```python
from build123d import *

# Parameters (mm, degrees)
F3_W         = 27
F3_H         = 27
F4_DEPTH     = 30
F5_T1_DEPTH  = 1002
F5_T3_DEPTH  = 1038
F5_T5_DEPTH  = 442
F5_T7_DEPTH  = 478
F5_T13_DEPTH = 447
F5_T17_DEPTH = 1007
F5_T20_DEPTH = 1012
F5_T22_DEPTH = 1050
F5_T24_DEPTH = 1005
F5_T26_DEPTH = 445
F5_T28_DEPTH = 490
F5_T30_DEPTH = 452
F5_T36_DEPTH = 1010
F5_T40_DEPTH = 450
F5_T47_DEPTH = 1010
F5_T51_DEPTH = 450


# Not quite as in the source:
# - a fillet or chamfer that OpenCascade refuses, or shapes differently, is made with other operations: its cross-section is extruded or revolved along the edge and cut away or added


with BuildPart() as f2:
    # F2: sweep along a path in F1
    with BuildLine(Plane.XY) as f2_path:
        Line((0, 0), (0, 440))
        Line((0, 440), (-1000, 440))
    # F0 (on Front) → F2 (sweep)
    with BuildSketch(Plane.XZ):
        Polygon((38, -2), (38, -25), (40, -25), (40, 0), (0, 0), (0, -350), (27, -350), (27, -376), (29, -376), (29, -348), (2, -348), (2, -2), align=None)
    sweep(path=f2_path.line, transition=Transition.RIGHT)

    # F3 (on face) → F4 (cut)
    with BuildSketch(Plane.XY.offset(-348)):
        with Locations((15.5, 455.5)):
            Rectangle(F3_W, F3_H)
    extrude(amount=-F4_DEPTH, mode=Mode.SUBTRACT)

    # F5: fillet of radius 2 on 15 edges, made by hand

    # F5_s2 → F5_t1 (join)
    with BuildSketch(Plane.YZ.offset(-1000)):
        with BuildLine():
            ThreePointArc((442, -346), (442.5857864376, -347.4142135624), (444, -348))
            Line((444, -348), (442, -348))
            Line((442, -348), (442, -346))
        make_face()
        with BuildLine():
            ThreePointArc((465, -350), (466.4142135624, -350.5857864376), (467, -352))
            Line((467, -352), (467, -350))
            Line((467, -350), (465, -350))
        make_face()
        with BuildLine():
            ThreePointArc((444, -2), (442.5857864376, -2.5857864376), (442, -4))
            Line((442, -4), (442, -2))
            Line((442, -2), (444, -2))
        make_face()
    extrude(amount=F5_T1_DEPTH)

    # F5_s4 → F5_t3 (join)
    with BuildSketch(Plane.YZ.offset(-1000)):
        with BuildLine():
            ThreePointArc((476, -2), (477.4142135624, -2.5857864376), (478, -4))
            Line((478, -4), (478, -2))
            Line((478, -2), (476, -2))
        make_face()
    extrude(amount=F5_T3_DEPTH)

    # F5_s6 → F5_t5 (join)
    with BuildSketch(Plane.XZ.offset(-442)):
        with BuildLine():
            ThreePointArc((25, -350), (26.4142135624, -350.5857864376), (27, -352))
            Line((27, -352), (27, -350))
            Line((27, -350), (25, -350))
        make_face()
        with BuildLine():
            ThreePointArc((4, -2), (2.5857864376, -2.5857864376), (2, -4))
            Line((2, -4), (2, -2))
            Line((2, -2), (4, -2))
        make_face()
    extrude(amount=F5_T5_DEPTH)

    # F5_s8 → F5_t7 (join)
    with BuildSketch(Plane.XZ.offset(-478)):
        with BuildLine():
            ThreePointArc((38, -4), (37.4142135624, -2.5857864376), (36, -2))
            Line((36, -2), (38, -2))
            Line((38, -2), (38, -4))
        make_face()
    extrude(amount=F5_T7_DEPTH)


with BuildPart() as f5_tool11:
    # F5_s12 → F5_t13 (new body)
    with BuildSketch(Plane.XZ):
        with BuildLine():
            ThreePointArc((4, -2), (2.5857864376, -2.5857864376), (2, -4))
            Line((2, -4), (2, -2))
            Line((2, -2), (4, -2))
        make_face()
    extrude(amount=-F5_T13_DEPTH)

    split(bisect_by=Plane.XZ.offset(-442), keep=Keep.BOTTOM)


with BuildPart() as f5_tool15:
    # F5_s16 → F5_t17 (new body)
    with BuildSketch(Plane.YZ.offset(7)):
        with BuildLine():
            ThreePointArc((444, -2), (442.5857864376, -2.5857864376), (442, -4))
            Line((442, -4), (442, -2))
            Line((442, -2), (444, -2))
        make_face()
    extrude(amount=-F5_T17_DEPTH)

    split(bisect_by=Plane.YZ.offset(2), keep=Keep.TOP)


with BuildPart() as f5_tool11_1:
    add(f5_tool11.part)

    # F5_t19: intersect F5_tool15
    add(f5_tool15.part, mode=Mode.INTERSECT)


with BuildPart() as f2_1:
    add(f2.part)

    # F5_t9: union F5_tool11
    add(f5_tool11_1.part)

    # F5_s21 → F5_t20 (cut)
    with BuildSketch(Plane.YZ.offset(-1005)):
        with BuildLine():
            ThreePointArc((467, -348), (468.4142135624, -348.5857864376), (469, -350))
            Line((469, -350), (469, -348))
            Line((469, -348), (467, -348))
        make_face()
    extrude(amount=F5_T20_DEPTH, mode=Mode.SUBTRACT)

    # F5_s23 → F5_t22 (cut)
    with BuildSketch(Plane.YZ.offset(-1005)):
        with BuildLine():
            ThreePointArc((480, -2), (479.4142135624, -0.5857864376), (478, 0))
            Line((478, 0), (480, 0))
            Line((480, 0), (480, -2))
        make_face()
    extrude(amount=F5_T22_DEPTH, mode=Mode.SUBTRACT)

    # F5_s25 → F5_t24 (cut)
    with BuildSketch(Plane.YZ.offset(-1005)):
        with BuildLine():
            ThreePointArc((440, -2), (440.5857864376, -0.5857864376), (442, 0))
            Line((442, 0), (440, 0))
            Line((440, 0), (440, -2))
        make_face()
        with BuildLine():
            ThreePointArc((440, -348), (440.5857864376, -349.4142135624), (442, -350))
            Line((442, -350), (440, -350))
            Line((440, -350), (440, -348))
        make_face()
    extrude(amount=F5_T24_DEPTH, mode=Mode.SUBTRACT)

    # F5_s27 → F5_t26 (cut)
    with BuildSketch(Plane.XZ.offset(-440)):
        with BuildLine():
            ThreePointArc((0, -2), (0.5857864376, -0.5857864376), (2, 0))
            Line((2, 0), (0, 0))
            Line((0, 0), (0, -2))
        make_face()
        with BuildLine():
            ThreePointArc((2, -350), (0.5857864376, -349.4142135624), (0, -348))
            Line((0, -348), (0, -350))
            Line((0, -350), (2, -350))
        make_face()
    extrude(amount=F5_T26_DEPTH, mode=Mode.SUBTRACT)

    # F5_s29 → F5_t28 (cut)
    with BuildSketch(Plane.XZ.offset(-485)):
        with BuildLine():
            ThreePointArc((38, 0), (39.4142135624, -0.5857864376), (40, -2))
            Line((40, -2), (40, 0))
            Line((40, 0), (38, 0))
        make_face()
    extrude(amount=F5_T28_DEPTH, mode=Mode.SUBTRACT)

    # F5_s31 → F5_t30 (cut)
    with BuildSketch(Plane.XZ.offset(-447)):
        with BuildLine():
            ThreePointArc((27, -348), (28.4142135624, -348.5857864376), (29, -350))
            Line((29, -350), (29, -348))
            Line((29, -348), (27, -348))
        make_face()
    extrude(amount=F5_T30_DEPTH, mode=Mode.SUBTRACT)


with BuildPart() as f5_tool34:
    # F5_s35 → F5_t36 (new body)
    with BuildSketch(Plane.YZ.offset(5)):
        with BuildLine():
            ThreePointArc((440, -2), (440.5857864376, -0.5857864376), (442, 0))
            Line((442, 0), (440, 0))
            Line((440, 0), (440, -2))
        make_face()
    extrude(amount=-F5_T36_DEPTH)

    split(bisect_by=Plane.YZ, keep=Keep.TOP)


with BuildPart() as f5_tool38:
    # F5_s39 → F5_t40 (new body)
    with BuildSketch(Plane.XZ.offset(5)):
        with BuildLine():
            ThreePointArc((0, -2), (0.5857864376, -0.5857864376), (2, 0))
            Line((2, 0), (0, 0))
            Line((0, 0), (0, -2))
        make_face()
    extrude(amount=-F5_T40_DEPTH)

    split(bisect_by=Plane.XZ.offset(-440), keep=Keep.BOTTOM)


with BuildPart() as f5_tool34_1:
    add(f5_tool34.part)

    # F5_t42: intersect F5_tool38
    add(f5_tool38.part, mode=Mode.INTERSECT)


with BuildPart() as f2_2:
    add(f2_1.part)

    # F5_t32: cut F5_tool34
    add(f5_tool34_1.part, mode=Mode.SUBTRACT)


with BuildPart() as f5_tool45:
    # F5_s46 → F5_t47 (new body)
    with BuildSketch(Plane.YZ.offset(5)):
        with BuildLine():
            ThreePointArc((440, -348), (440.5857864376, -349.4142135624), (442, -350))
            Line((442, -350), (440, -350))
            Line((440, -350), (440, -348))
        make_face()
    extrude(amount=-F5_T47_DEPTH)

    split(bisect_by=Plane.YZ, keep=Keep.TOP)


with BuildPart() as f5_tool49:
    # F5_s50 → F5_t51 (new body)
    with BuildSketch(Plane.XZ.offset(5)):
        with BuildLine():
            ThreePointArc((2, -350), (0.5857864376, -349.4142135624), (0, -348))
            Line((0, -348), (0, -350))
            Line((0, -350), (2, -350))
        make_face()
    extrude(amount=-F5_T51_DEPTH)

    split(bisect_by=Plane.XZ.offset(-440), keep=Keep.BOTTOM)


with BuildPart() as f5_tool45_1:
    add(f5_tool45.part)

    # F5_t53: intersect F5_tool49
    add(f5_tool49.part, mode=Mode.INTERSECT)


with BuildPart() as f2_3:
    add(f2_2.part)

    # F5_t43: cut F5_tool45
    add(f5_tool45_1.part, mode=Mode.SUBTRACT)


solid = f2_3.part
```
Can you work these out from the model? Positions are in its coordinate system, mm. A direction names the side the tool comes from. Give positions to 0.01 mm unless a question says otherwise; leave off trailing zeros. Loops run counter-clockwise (first coordinate to the right, second up) from the corner with the lowest first, then second, coordinate; pieces in that order, holes last. Notation, with made-up numbers: M 64.5,30.25 L 115.5,30.25 A18 ccw 115.5,44.25 Z; hole C 7.25,38.5 d7. An arc over 180 degrees is marked long. One line per item, written item: value.
(1) Suppose I cut it at B-B on y = 173. List the corners of the cut face in (x, z) for me, plus the area to 3 significant figures.
Returned:
outline: M 0,-348 A2 ccw 2,-350 L 25,-350 A2 cw 27,-352 L 27,-376 L 29,-376 L 29,-350 A2 ccw 27,-348 L 2,-348 L 2,-4 A2 cw 4,-2 L 36,-2 A2 cw 38,-4 L 38,-25 L 40,-25 L 40,-2 A2 ccw 38,0 L 2,0 A2 ccw 0,-2 Z
area: 927 mm^2
(2) Suppose I cut it at C-C on z = -115. List the corners of the cut face in (x, y) for me.
Returned:
outline: M -1000,440 L 0,440 L 0,0 L 2,0 L 2,442 L -1000,442 Z
(3) We'd pull the mould along Y, two halves only. Please class faces 4 (the face through (-506, 469, -363)), 5 (the face through (-507, 440, -173)), 6 (the face through (-331, 451, -2)): released by +Y, released by -Y, zero draft, split by the parting line, or undercut.
Returned:
face 4: released by +Y
face 5: released by -Y
face 6: undercut
(4) I need wall thicknesses on line 1 (Y direction, x = -848.5, z = -24); line 2 (X direction, y = 33, z = -200); line 3 (Y direction, x = -923, z = -173.5). Which ranges of each line are inside material? Lowest first, please.
Returned:
line 1: 440 to 442, 478 to 480
line 2: 0 to 2
line 3: 440 to 442
(5) Suppose I cut it at A-A on x = -371. List the corners of the cut face in (y, z) for me, plus the area to 3 significant figures.
Returned:
outline: M 440,-348 A2 ccw 442,-350 L 465,-350 A2 cw 467,-352 L 467,-376 L 469,-376 L 469,-350 A2 ccw 467,-348 L 444,-348 A2 cw 442,-346 L 442,-4 A2 cw 444,-2 L 476,-2 A2 cw 478,-4 L 478,-25 L 480,-25 L 480,-2 A2 ccw 478,0 L 442,0 A2 ccw 440,-2 Z
area: 928 mm^2
(6) Which directions (+Z, -Z, +X, -X, +Y, -Y) give clear straight access to the entire face, cutting with the end or side of a thin tool? Please do faces 1 (the face through (29, 224, -363)), 2 (the face through (-488, 478, -14)), 3 (the face through (-506, 467, -364)).
Returned:
face 1: -Z, +X, +Y, -Y
face 2: -Z, -X
face 3: -Z, +X, -X, -Y
(7) Will these pins go through, and if not, where does the flat tip stop? pin 1 (1 mm diameter, centred on x = -763, z = -138.5, fed in from +Y); pin 2 (10.5 mm diameter, centred on y = 323.5, z = -9.5, fed in from -X); pin 3 (5 mm diameter, centred on x = -780.5, z = -292, fed in from -Y); pin 4 (8 mm diameter, centred on x = 9, z = -362, fed in from +Y).
Returned:
pin 1: y = 442
pin 2: x = 0
pin 3: y = 440
pin 4: through
